Part model, mm, in its own coordinate system. A direction names the side the tool comes from. Coordinates: 2 decimals unless noted, no trailing zeros. Loops run counter-clockwise (first coordinate to the right, second up) from the corner with the lowest first, then second, coordinate; pieces in that order, holes last. Notation, with made-up numbers: (46, 36.5) -> (82, 36.5) arc R17 cw to (82, 64.5) -> close; hole circle Ø10 at (21.5, 50). An arc over 180 degrees is marked (long way). One line per item, written item: value. Start each with the question number.
from build123d import *

# Parameters (mm, degrees)
P_IDAT_VYSUNUT_M1_DEPTH  = 5.6
SKO_EPINA1_T             = 1.8
P_IDAT_VYSUNUT_M3_DEPTH  = 5.15
P_IDAT_VYSUNUT_M4_DEPTH  = 7.4
P_IDAT_VYSUNUT_M5_DEPTH  = 1.5
SKICA14_W                = 49.9
SKICA14_H                = 0.995009232
P_IDAT_VYSUNUT_M6_DEPTH  = 1.5
SKICA15_R                = 5.4
SKICA15_W                = 3
SKICA15_H                = 9
P_IDAT_VYSUNUT_M7_DEPTH  = 5.6
SKICA16_R                = 2
ODEBRAT_VYSUNUT_M1_DEPTH = 5.75
ZKOSEN_1_SIZE            = 1
SKICA17_W                = 24
SKICA17_H                = 13.4
ODEBRAT_VYSUNUT_M2_DEPTH = 1.6
ODEBRAT_VYSUNUT_M3_REACH = 442.031
SKICA23_R                = 2
ODEBRAT_VYSUNUT_M4_DEPTH = 5.7
SKICA24_R                = 2
ODEBRAT_VYSUNUT_M5_DEPTH = 5.7
SKICA25_R                = 6.25
ODEBRAT_VYSUNUT_M6_DEPTH = 1.5
SKICA26_W                = 214.14008497
SKICA26_H                = 14.05
ODEBRAT_VYSUNUT_M7_DEPTH = 443.82576223


with BuildPart() as part:
    # Skica3 → P_idat vysunut_m1 (new body)
    with BuildSketch(Plane.XY):
        Polygon((2.412545276, -4), (412.692715215, -4), (412.692715215, -118.191389918), (412.654731358, -118.229366948), (404.717731358, -118.229366948), (402.336688893, -120.609981536), (12.768122748, -120.609981536), (10.387229089, -118.22921813), (2.450229089, -118.22921813), (2.412545276, -118.191536378), align=None)
    extrude(amount=P_IDAT_VYSUNUT_M1_DEPTH)

    # Sko_epina1
    sko_epina1_openings = [part.faces().sort_by_distance(p)[0] for p in [
        (207.552632266, -62.25279763, 5.6),
    ]]
    offset(amount=SKO_EPINA1_T, openings=sko_epina1_openings, kind=Kind.INTERSECTION)



with BuildPart() as body_2:
    # Skica7 → P_idat vysunut_m3 (new body)
    with BuildSketch(Plane.XY.offset(5.6)):
        Polygon((-6.587454724, 5), (-6.587454724, -121.919602656), (-1.277548758, -127.22921813), (6.659451242, -127.22921813), (9.040344901, -129.609981536), (406.06413722, -129.609981536), (408.445179685, -127.229366948), (416.382179685, -127.229366948), (421.692715215, -121.919785731), (421.692715215, 5), align=None)
        Polygon((-3.787454724, 2.2), (-3.787454724, -120.759759814), (-0.11779565, -124.42921813), (7.81920435, -124.42921813), (10.200098009, -126.809981536), (404.904486629, -126.809981536), (407.285529094, -124.429366948), (415.222529094, -124.429366948), (418.892715215, -120.759840367), (418.892715215, 2.2), align=None, mode=Mode.SUBTRACT)
    extrude(amount=P_IDAT_VYSUNUT_M3_DEPTH)


with BuildPart() as part_1:
    add(part.part)

    add(body_2.part)  # P_idat vysunut_m4 merges body 2
    # Skica8 → P_idat vysunut_m4 (add)
    with BuildSketch(Plane(origin=(0, 0, 5.6), x_dir=(-1, 0, 0), z_dir=(0, 0, -1))):
        Polygon((-421.692715215, 5), (6.587454724, 5), (6.587454724, -121.919602656), (1.277548758, -127.22921813), (-6.659451242, -127.22921813), (-9.040344901, -129.609981536), (-406.06413722, -129.609981536), (-408.445179685, -127.229366948), (-416.382179685, -127.229366948), (-421.692715215, -121.919785731), align=None)
        Polygon((-0.612545276, -2.2), (-0.612545276, -118.937149634), (-1.70467352, -120.02921813), (-9.64167352, -120.02921813), (-12.022567179, -122.409981536), (-403.082178558, -122.409981536), (-405.463221024, -120.029366948), (-413.400221024, -120.029366948), (-414.492715215, -118.93706908), (-414.492715215, -2.2), align=None, mode=Mode.SUBTRACT)
    extrude(amount=P_IDAT_VYSUNUT_M4_DEPTH)

    # Skica11 → P_idat vysunut_m5 (add)
    with BuildSketch(Plane.XY.offset(10.75)):
        Polygon((421.692715215, 5), (-6.587454724, 5), (-6.587454724, -121.919602656), (-1.277548758, -127.22921813), (6.659451242, -127.22921813), (9.040344901, -129.609981536), (406.06413722, -129.609981536), (408.445179685, -127.229366948), (416.382179685, -127.229366948), (421.692715215, -121.919785731), align=None)
        Polygon((420.052630246, 3.195009232), (-4.947369754, 3.195009232), (-4.947369754, -120.114611888), (-0.239981646, -124.821742467), (7.697018354, -124.821742467), (10.68042987, -127.804990768), (404.42405225, -127.804990768), (406.805094715, -125.424376181), (414.742094715, -125.424376181), (420.052630246, -120.114794964), align=None, mode=Mode.SUBTRACT)
    extrude(amount=P_IDAT_VYSUNUT_M5_DEPTH)

    # Skica14 → P_idat vysunut_m6 (add)
    with BuildSketch(Plane.XY.offset(10.75)):
        with Locations((157.582630246, 2.697504616)):
            Rectangle(SKICA14_W, SKICA14_H)
        with Locations((257.522630246, 2.697504616)):
            Rectangle(SKICA14_W, SKICA14_H)
        with Locations((257.52224106, -127.307486152)):
            Rectangle(SKICA14_W, SKICA14_H)
        with Locations((157.58224106, -127.307486152)):
            Rectangle(SKICA14_W, SKICA14_H)
    extrude(amount=P_IDAT_VYSUNUT_M6_DEPTH)

    # Skica15 → P_idat vysunut_m7 (add)
    with BuildSketch(Plane.XY):
        with Locations((3.968545276, -115.95421813)):
            Circle(SKICA15_R)
        with Locations((33.491545276, -69.050981536)):
            Circle(SKICA15_R)
        with Locations((411.197715215, -115.879366948)):
            Circle(SKICA15_R)
        with Locations((334.147715215, -53.972)):
            Circle(SKICA15_R)
        with Locations((36.401545276, 0)):
            Rectangle(SKICA15_W, SKICA15_H)
    extrude(amount=P_IDAT_VYSUNUT_M7_DEPTH)

    # Skica16 → Odebrat vysunut_m1 (cut)
    with BuildSketch(Plane.XY.offset(5.6)):
        with Locations((3.968545276, -115.95421813)):
            Circle(SKICA16_R)
        with Locations((33.491545276, -69.050981536)):
            Circle(SKICA16_R)
        with Locations((334.147715215, -53.972)):
            Circle(SKICA16_R)
        with Locations((411.197715215, -115.879366948)):
            Circle(SKICA16_R)
    extrude(amount=-ODEBRAT_VYSUNUT_M1_DEPTH, mode=Mode.SUBTRACT)

    # Zkosen_1
    zkosen_1_edges = [part_1.edges().sort_by_distance(p)[0] for p in [
        (8.049207709, -112.417525591, 0),
        (28.091545276, -69.050981536, 0),
        (407.069426922, -112.398384936, 0),
        (328.747715215, -53.972, 0),
    ]]
    chamfer(zkosen_1_edges, length=ZKOSEN_1_SIZE)

    # Skica17 → Odebrat vysunut_m2 (cut)
    with BuildSketch(Plane.XY.offset(5.6)):
        with Locations((36.401545276, -4.5)):
            Rectangle(SKICA17_W, SKICA17_H)
    extrude(amount=-ODEBRAT_VYSUNUT_M2_DEPTH, mode=Mode.SUBTRACT)

    # Odebrat vysunut_m3: up to this face of the body (flat: up to its plane)
    odebrat_vysunut_m3_end = Plane(part_1.part.faces().sort_by_distance((207.552630246, 5, 5.225))[0])
    # Skica18 → Odebrat vysunut_m3 (cut, up to the picked face)
    with BuildSketch(Plane.XZ.offset(4.5), mode=Mode.PRIVATE) as odebrat_vysunut_m3_sk1:
        with BuildLine():
            Line((33.651545276, 7.5), (39.151545276, 7.5))
            ThreePointArc((39.151545276, 7.5), (42.651545276, 4), (39.151545276, 0.5))
            Line((39.151545276, 0.5), (33.651545276, 0.5))
            ThreePointArc((33.651545276, 0.5), (30.151545276, 4), (33.651545276, 7.5))
        make_face()
    odebrat_vysunut_m3_tool1 = split(extrude(odebrat_vysunut_m3_sk1.sketch, amount=-ODEBRAT_VYSUNUT_M3_REACH, mode=Mode.PRIVATE), bisect_by=odebrat_vysunut_m3_end, keep=Keep.BOTH, mode=Mode.PRIVATE)
    add(odebrat_vysunut_m3_tool1.solids().sort_by(Axis((36.401545, -4.5, 4), (0, 1, 0)))[0], mode=Mode.SUBTRACT)

    # Skica23 → Odebrat vysunut_m4 (cut)
    with BuildSketch(Plane.ZY.offset(6.587454724)):
        with Locations((3.2, -18.459801328)):
            Circle(SKICA23_R)
        with Locations((3.2, -98.459801328)):
            Circle(SKICA23_R)
    extrude(amount=-ODEBRAT_VYSUNUT_M4_DEPTH, mode=Mode.SUBTRACT)

    # Skica24 → Odebrat vysunut_m5 (cut)
    with BuildSketch(Plane(origin=(421.692715215, 0, 0), x_dir=(0, 0, -1), z_dir=(1, 0, 0))):
        with Locations((-3.2, -18.459892866)):
            Circle(SKICA24_R)
        with Locations((-3.2, -98.459892866)):
            Circle(SKICA24_R)
    extrude(amount=-ODEBRAT_VYSUNUT_M5_DEPTH, mode=Mode.SUBTRACT)

    # Skica25 → Odebrat vysunut_m6 (cut)
    with BuildSketch(Plane(origin=(0, 0, -1.8), x_dir=(-1, 0, 0), z_dir=(0, 0, -1))):
        with Locations((-401.692715215, -15)):
            Circle(SKICA25_R)
        with Locations((-13.412545276, -15)):
            Circle(SKICA25_R)
        with Locations((-388.445179685, -109.609981536)):
            Circle(SKICA25_R)
        with Locations((-26.659451242, -109.609981536)):
            Circle(SKICA25_R)
    extrude(amount=-ODEBRAT_VYSUNUT_M6_DEPTH, mode=Mode.SUBTRACT)

    # Skica26 → Odebrat vysunut_m7 (cut, through all)
    with BuildSketch(Plane(origin=(0, 5, 0), x_dir=(1, 0, 0), z_dir=(0, 1, 0))):
        with Locations((100.482587761, -5.225)):
            Rectangle(SKICA26_W, SKICA26_H)
    extrude(amount=-ODEBRAT_VYSUNUT_M7_DEPTH, mode=Mode.SUBTRACT)


solid = part_1.part
1) Slice it at B-B (x = 225). Give the cut face in (y, z) (3 decimals).
2) Pull direction Z, two halves, no side cores. Call faces 4 (the cylindrical face through (336.639, -58.763, 3.268)), 5 (the cylindrical face through (418.883, -16.773, 2.125)), 6 (the flat face through (411, -116, -0.15)): +Z half, -Z half, draft (parallel to the pull), parting line (faces both ways), or undercut.
3) Slice it at A-A (y = -70). Give the cut face in (x, z).
4) Probe line 1 (Y direction, x = 249.5, z = 11); line 2 (Y direction, x = 341, z = 2.5); line 3 (Y direction, x = 333.5, z = 3.75). List the from-to ranges inside material, lowest first. Write a range as from..to.
5) Pin check, flat tips, straight feed: pin 1 Ø1 at (y, z) = (-71.5, 5.5) entering from -X; pin 2 Ø2 at (y, z) = (-18.5, 3) entering from +X; pin 3 Ø4 at (x, y) = (380.5, -95.5) entering from +Z. Stop position of each tip, or through.
6) Tool access for faces 1 (the flat face through (412, -127.229, 5)), 2 (the cylindrical face through (332.56, -55.19, 2.77)), 3 (the flat face through (389, -110, -0.3)): list every direction of +Z, -Z, +X, -X, +Y, -Y with a clear straight run to the whole face (end or side of a thin tool).
7) Slice it at C-C (z = 8.25). Give the cut face in (x, y), then the cut area to 3 significant figures.
Check sheet entries:
1. outline: (-129.61, -1.8) -> (5, -1.8) -> (5, 12.25) -> (3.195, 12.25) -> (3.195, 10.75) -> (2.2, 10.75) -> (2.2, 5.6) -> (-4, 5.6) -> (-4, 0) -> (-120.61, 0) -> (-120.61, 5.6) -> (-126.81, 5.6) -> (-126.81, 10.75) -> (-127.805, 10.75) -> (-127.805, 12.25) -> (-129.61, 12.25) -> close
2. face 4: draft
2. face 5: undercut
2. face 6: +Z half
3. outline: (207.55, -1.8) -> (421.69, -1.8) -> (421.69, 12.25) -> (420.05, 12.25) -> (420.05, 10.75) -> (418.89, 10.75) -> (418.89, 5.6) -> (412.69, 5.6) -> (412.69, 0) -> (207.55, 0) -> close
4. line 1: y = -129.61..-126.81, 2.2..5
4. line 2: y = -129.61..-120.61, -4..5
4. line 3: y = -129.61..-120.61, -59.33..-55.86, -52.08..-48.61, -4..5
5. pin 1: stops at x = 412.69
5. pin 2: stops at x = 415.99
5. pin 3: stops at z = 0
6. face 1: +Z, -Z, +X, -Y
6. face 2: +Z
6. face 3: -Z
7. outline: (207.55, -129.61) -> (406.06, -129.61) -> (408.45, -127.23) -> (416.38, -127.23) -> (421.69, -121.92) -> (421.69, 5) -> (207.55, 5) -> (207.55, 2.2) -> (418.89, 2.2) -> (418.89, -120.76) -> (415.22, -124.43) -> (407.29, -124.43) -> (404.9, -126.81) -> (207.55, -126.81) -> close
7. area: 1,550 mm^2
